Geometry: final body of the model. Coordinates: model frame, mm. Coordinates: 2 decimals unless noted, no trailing zeros. Loops run counter-clockwise (first coordinate to the right, second up) from the corner with the lowest first, then second, coordinate; pieces in that order, holes last. Notation, with made-up numbers: (79, 32.25) - (120, 32.25) arc R17 cw to (120, 45.25) - close; hole circle Ø10 at (84.25, 56). An arc over 180 degrees is marked (long way). Return JSON: item names as keys, results as strings.
from build123d import *

# Parameters (mm, degrees)
SKETCH_1_R      = 140
SKETCH_1_R_2    = 35
SKETCH_1_R_3    = 1.75
SKETCH_1_R_4    = 5
EXTRUDE_1_DEPTH = 10


with BuildPart() as part:
    # 草图1 → 凸台-拉伸1 (new body)
    with BuildSketch(Plane(origin=(0, 0, 0), x_dir=(0, 0, -1), z_dir=(1, 0, 0))):
        with Locations((-24.920952127, 0.093336899)):
            Circle(SKETCH_1_R)
        with Locations((-24.920952127, 0.093336899)):
            Circle(SKETCH_1_R_2, mode=Mode.SUBTRACT)
        with Locations((-24.920952127, 42.593336899)):
            Circle(SKETCH_1_R_3, mode=Mode.SUBTRACT)
        with Locations((5.131086073, 30.1453751)):
            Circle(SKETCH_1_R_3, mode=Mode.SUBTRACT)
        with Locations((17.579047873, 0.093336899)):
            Circle(SKETCH_1_R_3, mode=Mode.SUBTRACT)
        with Locations((5.131086073, -29.958701301)):
            Circle(SKETCH_1_R_3, mode=Mode.SUBTRACT)
        with Locations((-24.920952127, -42.406663101)):
            Circle(SKETCH_1_R_3, mode=Mode.SUBTRACT)
        with Locations((-54.972990328, -29.958701301)):
            Circle(SKETCH_1_R_3, mode=Mode.SUBTRACT)
        with Locations((-67.420952127, 0.093336899)):
            Circle(SKETCH_1_R_3, mode=Mode.SUBTRACT)
        with Locations((-54.972990328, 30.1453751)):
            Circle(SKETCH_1_R_3, mode=Mode.SUBTRACT)
        with Locations((-149.920952127, 0.093336899)):
            Circle(SKETCH_1_R_4, mode=Mode.SUBTRACT)
        with Locations((-24.920952127, 125.093336899)):
            Circle(SKETCH_1_R_4, mode=Mode.SUBTRACT)
        with Locations((100.079047873, 0.093336899)):
            Circle(SKETCH_1_R_4, mode=Mode.SUBTRACT)
        with Locations((-24.920952127, -124.906663101)):
            Circle(SKETCH_1_R_4, mode=Mode.SUBTRACT)
    extrude(amount=EXTRUDE_1_DEPTH)


solid = part.part
Item 1: Section query B-B, the plane x = 7.25. Count the separate pieces of the cut face and the enclosed holes in it, and give its area (3 significant figures).
Worked out:
{"separate pieces": "1", "enclosed holes": "13", "area": "57,300 mm^2"}
Item 2: Ray query, probe 1 along Z at (x, y) = (1, -30); probe 2 along Y at (x, z) = (6.75, 151); probe 3 along Y at (x, z) = (0.5, 68.5). Return the intervals inside material, ascending. Write a range as from..to.
Worked out:
{"probe 1": "-111.81..-6.88, -3.38..7.05, 42.79..53.22, 56.72..161.65", "probe 2": "-60.77..-4.79, 4.98..60.95", "probe 3": "-132.95..-1.28, 1.47..133.14"}
Item 3: Section query C-C, the plane z = -63. Return loops of the section in (x, y).
Worked out:
{"outline": "(0, -108.86) - (10, -108.86) - (10, 109.04) - (0, 109.04) - close"}
Item 4: Section query A-A, the plane y = 24. Return loops of the section in (x, z), and give its area (3 significant figures).
Worked out:
{"outline": "(0, -113.02) - (10, -113.02) - (10, -0.64) - (0, -0.64) - close; (0, 50.48) - (10, 50.48) - (10, 162.86) - (0, 162.86) - close", "area": "2,250 mm^2"}
Item 5: First-contact query: pin 1 Ø4.5 at (y, z) = (30.15, -5.13) entering from +X; pin 2 Ø1.5 at (x, y) = (5, -83.5) entering from +Z; pin 3 Ø6 at (x, z) = (3.5, -86) entering from -Y; pin 4 Ø6 at (x, y) = (2.5, 112) entering from -Z. Flat tips, straight axial feed; report the tip coordinate or a pass-through.
Worked out:
{"pin 1": "x = 10", "pin 2": "z = 137.78", "pin 3": "y = -89.09", "pin 4": "z = -63.05"}
Item 6: Section query D-D, the plane y = 109. Return loops of the section in (x, z), and give its area (3 significant figures).
Worked out:
{"outline": "(0, -63.05) - (10, -63.05) - (10, 112.89) - (0, 112.89) - close", "area": "1,760 mm^2"}
